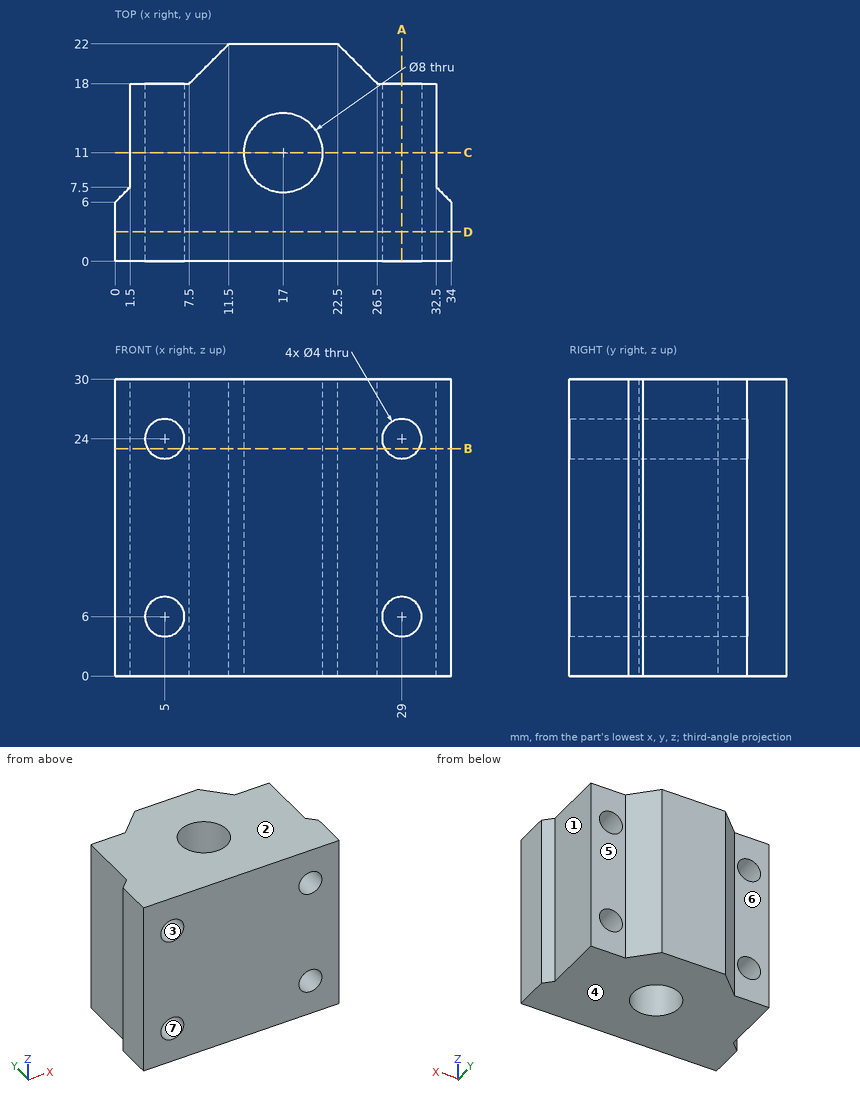
Check sheet for the drawn part. Datum: minimum x, y, z corner. Units: mm. A direction names the side the tool comes from. Give positions to 0.01 mm unless a question says otherwise; leave off trailing zeros. Write each loop counter-clockwise with the first axis right and the second up, starting at its lowest first coordinate (ties: lowest second). Pieces come first, ordered by that corner, then holes. Notation, with made-up numbers: (8.25, -38.75) - (64.25, -38.75) arc R33 cw to (64.25, -9.75) - close; hole circle Ø10 at (32.25, 79). An arc over 180 degrees is marked (long way). Put each result on its own line as item: value.
1. Sectioned sample at D-D, the plane y = 3. Enter the section's corners in (x, z), plus the area to 3 significant figures.
Ans:
outline: (0, 0) - (34, 0) - (34, 30) - (0, 30) - close; hole circle Ø4 at (5, 6); hole circle Ø4 at (5, 24); hole circle Ø4 at (29, 6); hole circle Ø4 at (29, 24)
area: 970 mm²
2. Thickness scan on line 1 (Y direction, x = 17, z = 10); line 2 (X direction, y = 8, z = 24); line 3 (Y direction, x = 32, z = 5.5). Record the ranges inside material, lowest first.
Ans:
line 1: y = 0 to 7, 15 to 22
line 2: x = 1.5 to 3, 7 to 14.35, 19.65 to 27, 31 to 32.5
line 3: y = 0 to 18
3. Go/stop test with flat-tipped pins: pin 1 (3 mm diameter, centred on x = 5, z = 15.5, fed in from +Y); pin 2 (4 mm diameter, centred on y = 8.5, z = 17, fed in from +X); pin 3 (11.5 mm diameter, centred on y = 14.5, z = 20.5, fed in from -X). Record where each tip stops, or that it passes through.
Ans:
pin 1: stops at y = 18
pin 2: stops at x = 33.5
pin 3: stops at x = 1.5
4. Sectioned sample at B-B, the plane z = 23. Enter the section's corners in (x, y).
Ans:
outline: (0, 0) - (3.27, 0) - (3.27, 18) - (1.5, 18) - (1.5, 7.5) - (0, 6) - close; (6.73, 0) - (27.27, 0) - (27.27, 18) - (26.5, 18) - (22.5, 22) - (11.5, 22) - (7.5, 18) - (6.73, 18) - close; (30.73, 0) - (34, 0) - (34, 6) - (32.5, 7.5) - (32.5, 18) - (30.73, 18) - close; hole circle Ø8 at (17, 11)
5. Set-up check for the marked faces 5, 6 and 7: record each of +Z, -Z, +X, -X, +Y, -Y from which the full face is reachable in a straight line by a thin tool's end or side.
Ans:
face 5: +Z, -Z, +X, +Y
face 6: +Z, -Z, -X, +Y
face 7: +Y, -Y
6. Sectioned sample at C-C, the plane y = 11. Enter the section's corners in (x, z), plus the area to 3 significant figures.
Ans:
outline: (1.5, 0) - (13, 0) - (13, 30) - (1.5, 30) - close; (21, 0) - (32.5, 0) - (32.5, 30) - (21, 30) - close; hole circle Ø4 at (5, 6); hole circle Ø4 at (5, 24); hole circle Ø4 at (29, 6); hole circle Ø4 at (29, 24)
area: 640 mm²
7. Draft check along Z on the marked faces 1, 2, 3 and 4. Enter one of: +Z half, -Z half, draft (parallel to the pull), parting line (faces both ways), or undercut.
Ans:
face 1: draft
face 2: +Z half
face 3: undercut
face 4: -Z half
8. Sectioned sample at A-A, the plane x = 29. Enter the section's corners in (y, z).
Ans:
outline: (0, 0) - (18, 0) - (18, 4) - (0, 4) - close; (0, 8) - (18, 8) - (18, 22) - (0, 22) - close; (0, 26) - (18, 26) - (18, 30) - (0, 30) - close
